Here's the drawing with two shaded views (mm, measured from the low corner). I have some questions. A direction names the side the tool comes from. Coordinates: 2 decimals unless noted, no trailing zeros. Write each loop counter-clockwise with the first axis right and the second up, starting at its lowest first coordinate (ties: lowest second). Pieces come first, ordered by that corner, then holes.
Item 1: If I drill on line 1 (Y direction, x = 1, z = 7.25); line 2 (Z direction, x = 3.5, y = 3.7); line 3 (Z direction, x = 1.25, y = 2.55), over which ranges is the centre line in solid material (lowest first)?
Item 2: If we section it at B-B (z = 2.75): Please give me the cut outline in (x, y).
Item 3: For the marked faces 1, 2 and 3, which set-ups out of +Z, -Z, +X, -X, +Y, -Y let a thin tool reach every point of the face, with its end or its side?
Item 4: If we section it at C-C (y = 1.85): Please give me the cut outline in (x, z).
Item 5: If we section it at A-A (x = 3.5): Please give me the cut outline in (y, z), then the cut area to 3 significant figures.
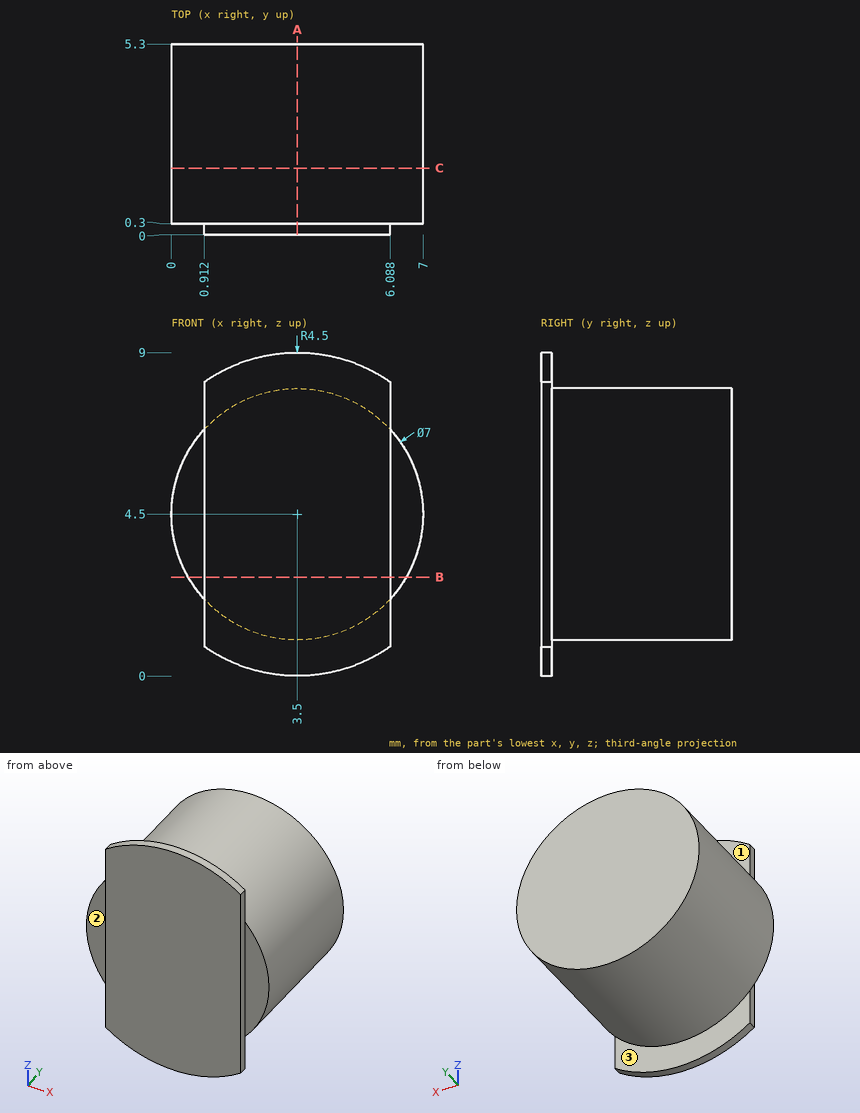
Answer list:
1. line 1: y = 0 to 0.3
1. line 2: z = 1 to 8
1. line 3: z = 1.82 to 7.18
2. outline: (0.47, 0.3) - (0.91, 0.3) - (0.91, 0) - (6.09, 0) - (6.09, 0.3) - (6.53, 0.3) - (6.53, 5.3) - (0.47, 5.3) - close
3. face 1: +Z, +Y
3. face 2: +Z, -Z, -X, -Y
3. face 3: -Z, +Y
4. outline: circle Ø7 at (3.5, 4.5)
5. outline: (0, 0) - (0.3, 0) - (0.3, 1) - (5.3, 1) - (5.3, 8) - (0.3, 8) - (0.3, 9) - (0, 9) - close
5. area: 37.7 mm2
